Input: part model. Units: mm. Frame: model coordinates. A direction names the side the tool comes from. Coordinates: 2 decimals unless noted, no trailing zeros. Write each loop counter-clockwise with the first axis right and the second up, starting at its lowest first coordinate (ties: lowest second). Pieces come first, ordered by that corner, then holes. Notation, with made-up numbers: M -33,17.5 L 13,17.5 A19 ccw 13,35.5 Z; hole C 8.5,47 d11. An arc over 180 degrees is marked long. Use one line per item in the form item = value.
from build123d import *

# Parameters (mm, degrees)
BOSS_EXTRUDE1_START = -5.08
SKETCH2_R           = 35.56
BOSS_EXTRUDE1_DEPTH = 5.08
SKETCH3_R           = 8.89
SKETCH3_R_2         = 6.35
SKETCH5_R           = 6.35
CUT_EXTRUDE1_DEPTH  = 146.358143907
SKETCH6_R           = 6.35
CUT_EXTRUDE2_DEPTH  = 142.398403103
SKETCH7_W           = 43.18
SKETCH7_H           = 76.2
CUT_EXTRUDE3_DEPTH  = 5.08
FILLET1_R           = 5.08


with BuildPart() as part:
    # Sketch1 → Revolve1 (revolve)
    with BuildSketch(Plane.XY, mode=Mode.PRIVATE) as revolve1_sk:
        Polygon((0, 0), (63.5, 0), (63.5, 76.2), (48.26, 76.2), (48.26, 127), (35.56, 127), (35.56, 63.5), (50.8, 63.5), (50.8, 12.7), (0, 12.7), align=None)
    revolve(revolve1_sk.sketch.rotate(Axis((0, 0, 0), (0, 1, 0)), 90), axis=Axis((0, 0, 0), (0, 1, 0)))

    # Sketch2 → Boss-Extrude1 (add)
    with BuildSketch(Plane(origin=(0, 114.3, 0), x_dir=(1, 0, 0), z_dir=(0, 1, 0)).offset(BOSS_EXTRUDE1_START)):
        with Locations(Location((0, 0, 0), (0, 0, 90))):
            Circle(SKETCH2_R)
    extrude(amount=BOSS_EXTRUDE1_DEPTH)

    # Sweep1: sweep along a path in Sketch4
    with BuildLine(Plane.XY) as sweep1_path:
        Line((15.24, 114.3), (15.24, 50.8))
        Line((15.24, 50.8), (33.02, 50.8))
        Line((33.02, 50.8), (33.02, 12.7))
    # Sketch3 → Sweep1 (sweep)
    with BuildSketch(Plane(origin=(0, 114.3, 0), x_dir=(1, 0, 0), z_dir=(0, 1, 0))):
        with Locations((15.24, 0)):
            Circle(SKETCH3_R)
        with Locations((15.24, 0)):
            Circle(SKETCH3_R_2, mode=Mode.SUBTRACT)
    sweep1 = sweep(path=sweep1_path.line, transition=Transition.RIGHT)

    # Sketch5 → Cut-Extrude1 (cut, through all)
    with BuildSketch(Plane(origin=(0, 12.7, 0), x_dir=(1, 0, 0), z_dir=(0, 1, 0))):
        with Locations((33.02, 0)):
            Circle(SKETCH5_R)
    cut_extrude1 = extrude(amount=-CUT_EXTRUDE1_DEPTH, mode=Mode.SUBTRACT)

    # Sketch6 → Cut-Extrude2 (cut, through all)
    with BuildSketch(Plane.XZ.offset(-109.22)):
        with Locations(Location((15.24, 0, 0), (0, 0, 90))):
            Circle(SKETCH6_R)
    cut_extrude2 = extrude(amount=-CUT_EXTRUDE2_DEPTH, mode=Mode.SUBTRACT)

    # Mirror1: Sweep1, Cut-Extrude1, Cut-Extrude2 across plane
    add(sweep1.mirror(Plane(origin=(0, 0, 0), x_dir=(0, 0, 1), z_dir=(1, 0, 0))))
    add(cut_extrude1.mirror(Plane(origin=(0, 0, 0), x_dir=(0, 0, 1), z_dir=(1, 0, 0))), mode=Mode.SUBTRACT)
    add(cut_extrude2.mirror(Plane(origin=(0, 0, 0), x_dir=(0, 0, 1), z_dir=(1, 0, 0))), mode=Mode.SUBTRACT)

    # Sketch7 → Cut-Extrude3 (cut)
    with BuildSketch(Plane.XY.offset(63.5)):
        with Locations((0, 38.1)):
            Rectangle(SKETCH7_W, SKETCH7_H)
    cut_extrude3 = extrude(amount=-CUT_EXTRUDE3_DEPTH, mode=Mode.SUBTRACT)

    # Mirror2: Cut-Extrude3 across plane
    add(cut_extrude3.mirror(Plane.XY), mode=Mode.SUBTRACT)

    # Fillet1
    fillet1_edges = [part.edges().sort_by_distance(p)[0] for p in [
        (0, 76.2, 48.26),
        (0, 114.3, 35.56),
    ]]
    fillet(fillet1_edges, radius=FILLET1_R)


solid = part.part
(1) Line query: probe 1 along X at (y, z) = (22, 0); probe 2 along Y at (x, z) = (15, -14.5); probe 3 along Y at (x, z) = (46, 8). Output: solid intervals per line, ascending.
Computed:
probe_1 = -63.5 to -50.8, -41.91 to -39.37, -26.67 to -24.13, 24.13 to 26.67, 39.37 to 41.91, 50.8 to 63.5
probe_2 = 0 to 12.7, 109.22 to 114.3
probe_3 = 0 to 12.7, 63.5 to 127
(2) Set-up query: faces 1 (the cylindrical face through (18.236, 78.886, 5.599)), 2 (the cylindrical face through (39.077, 22.625, -1.907)), 3 (the cylindrical face through (-6.36, 82.57, 0.39)). Return all of +Z, -Z, +X, -X, +Y, -Y with unobstructed straight access to the full face (end or side cutting, diameter ignored); none if empty.
Computed:
face_1 = +Y
face_2 = -Y
face_3 = none
(3) First-contact query: pin 1 Ø8 at (x, y) = (47, 86) entering from +Z; pin 2 Ø3 at (y, z) = (79.5, -10.5) entering from -X; pin 3 Ø3 at (y, z) = (49.5, 16) entering from +X. Flat tips, straight axial feed; report the tip coordinate or a pass-through.
Computed:
pin_1 = 21.91
pin_2 = -48.37
pin_3 = 61.82
(4) Pull-direction query (Z, two-part tool) for faces 4 (the cylindrical face through (24.34, 45.76, -3.86)), 5 (the flat face through (0, 39, -58.42)), 6 (the flat face through (9, 76.2, 53)), 7 (the cylindrical face through (-14.5, 104.46, -46.03)); classes: pulls with the +Z half, pulls with the -Z half, needs draft (parallel to the pull), parting line crosses it, or undercut.
Computed:
face_4 = undercut
face_5 = pulls with the -Z half
face_6 = needs draft
face_7 = parting line crosses it
(5) Section query C-C on y = 101. Return the cut outline in (x, z).
Computed:
outline = C 0,0 d96.52; C -15.24,0 d17.78; C 15.24,0 d17.78; hole C 0,0 d71.12; hole C -15.24,0 d12.7; hole C 15.24,0 d12.7
(6) Section query B-B on y = 71. Return the cut outline in (x, z).
Computed:
outline = C -15.24,0 d17.78; M -21.59,-59.72 L -21.59,-58.42 L 21.59,-58.42 L 21.59,-59.72 A63.5 ccw 21.59,59.72 L 21.59,58.42 L -21.59,58.42 L -21.59,59.72 A63.5 ccw Z; C 15.24,0 d17.78; hole C 0,0 d71.12; hole C -15.24,0 d12.7; hole C 15.24,0 d12.7
(7) Section query A-A on y = 50.8. Return the cut outline in (x, z).
Computed:
outline = M -33.02,-8.89 L -15.24,-8.89 A8.89 ccw -15.24,8.89 L -33.02,8.89 A8.89 ccw Z; M -21.59,-59.72 L -21.59,-58.42 L 21.59,-58.42 L 21.59,-59.72 A63.5 ccw 21.59,59.72 L 21.59,58.42 L -21.59,58.42 L -21.59,59.72 A63.5 ccw Z; M 15.24,-8.89 L 33.02,-8.89 A8.89 ccw 33.02,8.89 L 15.24,8.89 A8.89 ccw Z; hole C 0,0 d101.6; hole M -33.02,-6.35 L -15.24,-6.35 A6.35 ccw -15.24,6.35 L -33.02,6.35 A6.35 ccw Z; hole M 15.24,-6.35 L 33.02,-6.35 A6.35 ccw 33.02,6.35 L 15.24,6.35 A6.35 ccw Z
